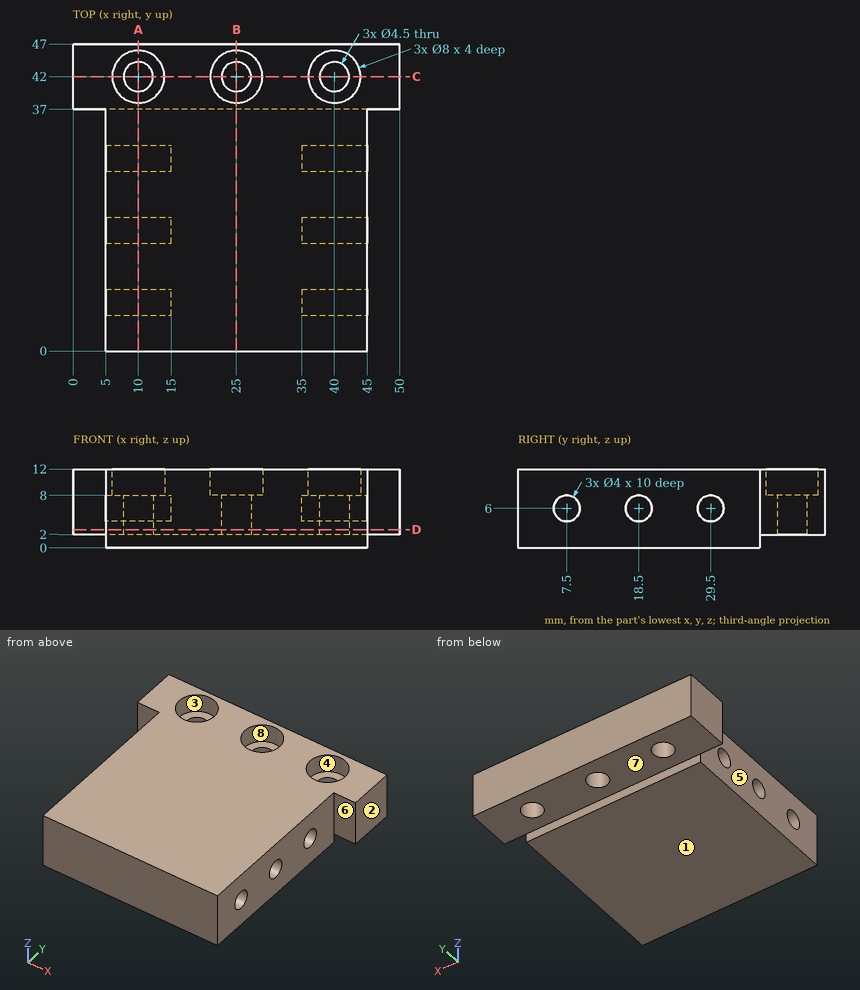
For this review, use the dimensioned drawing (mm, ordinates from the lowest corner) and the shaded views. A direction names the side the tool comes from. Round coordinates to 2 decimals unless told otherwise and drop trailing zeros. Write each loop counter-clockwise with the first axis right and the second up, starting at its lowest first coordinate (ties: lowest second). Pieces come first, ordered by that corner, then holes. Notation, with made-up numbers: (89, -39.75) - (105, -39.75) arc R19 ccw to (105, -29.75) - close; hole circle Ø11 at (0, 35). An arc over 180 degrees is marked (long way). One line per item, written item: value. Start each with the question number.
1. Machinability: for the marked faces 5, 6, 7 and 8, which of the approach directions +Z, -Z, +X, -X, +Y, -Y give a long, thin tool a straight path to every point of the face, cutting with its end or side? Answer none if there is none.
2. Consider section A-A on x = 10. Write out the cut boundary in (y, z), and give its area (3 significant figures).
3. Consider section B-B on x = 25. Write out the cut boundary in (y, z), and give its area (3 significant figures).
4. Consider section D-D on z = 2.75. Write out the cut boundary in (x, y), and give its area (3 significant figures).
5. Clearance check with flat-ended pins moving along their axes: P1, Ø1, axis at x = 18, z = 1, coming from the +Y side; P2, Ø2.5, axis at x = 27, y = 41.5, coming from the +Z side; P3, Ø6.5, axis at y = 7.5, z = 6, coming from the -X side. State where each tip first meets the part, or that it passes through.
6. Consider section C-C on y = 42. Write out the cut boundary in (x, z), and give its area (3 significant figures).
7. The part is to be moulded in two halves that separate along X. For the marked faces 1, 2, 3 and 4, say which applies: released by +X, released by -X, zero draft, split by the parting line, or undercut.
8. To check wall thickness, follow L1, parallel to Y at x = 40, z = 5.25; L2, parallel to Y at x = 25, z = 9.1; L3, parallel to Y at x = 42, z = 6. State the ranges of each line that lie inside material, in increasing order. Write a range as from..to.
Checks:
1. face 5: +Z, -Z, -X, -Y
1. face 6: +Z, -Z, +X, -Y
1. face 7: -Z, +X, -X, +Y
1. face 8: +Z
2. outline: (0, 0) - (37, 0) - (37, 2) - (39.75, 2) - (39.75, 8) - (38, 8) - (38, 12) - (0, 12) - close; (44.25, 2) - (47, 2) - (47, 12) - (46, 12) - (46, 8) - (44.25, 8) - close; hole circle Ø4 at (7.5, 6); hole circle Ø4 at (18.5, 6); hole circle Ø4 at (29.5, 6)
2. area: 447 mm^2
3. outline: (0, 0) - (37, 0) - (37, 2) - (39.75, 2) - (39.75, 8) - (38, 8) - (38, 12) - (0, 12) - close; (44.25, 2) - (47, 2) - (47, 12) - (46, 12) - (46, 8) - (44.25, 8) - close
3. area: 485 mm^2
4. outline: (0, 37) - (5, 37) - (5, 0) - (45, 0) - (45, 37) - (50, 37) - (50, 47) - (0, 47) - close; hole circle Ø4.5 at (10, 42); hole circle Ø4.5 at (25, 42); hole circle Ø4.5 at (40, 42)
4. area: 1,930 mm^2
5. P1: stops at y = 37
5. P2: stops at z = 8
5. P3: stops at x = 5
6. outline: (0, 2) - (7.75, 2) - (7.75, 8) - (6, 8) - (6, 12) - (0, 12) - close; (12.25, 2) - (22.75, 2) - (22.75, 8) - (21, 8) - (21, 12) - (14, 12) - (14, 8) - (12.25, 8) - close; (27.25, 2) - (37.75, 2) - (37.75, 8) - (36, 8) - (36, 12) - (29, 12) - (29, 8) - (27.25, 8) - close; (42.25, 2) - (50, 2) - (50, 12) - (44, 12) - (44, 8) - (42.25, 8) - close
6. area: 323 mm^2
7. face 1: zero draft
7. face 2: released by +X
7. face 3: undercut
7. face 4: undercut
8. L1: y = 0..5.65, 9.35..16.65, 20.35..27.65, 31.35..39.75, 44.25..47
8. L2: y = 0..38, 46..47
8. L3: y = 0..5.5, 9.5..16.5, 20.5..27.5, 31.5..40.97, 43.03..47
